Model file for the job. Use its own axes, mm. A direction names the side the tool comes from. Round coordinates to 2 decimals unless told otherwise and drop trailing zeros. Order: outer loops, then holes, each group sorted by start corner. A loop starts at its lowest first (then second) coordinate and runs counter-clockwise, first axis right, second up. Notation, with made-up numbers: (61.25, 68.25) - (120.25, 68.25) arc R18 cw to (120.25, 76.25) - close; hole circle Ø9 at (-37.75, -4.75). An arc over 180 degrees is marked (long way). Put each result on its own line as item: value. Start each with the question number.
Item 1: Which spindle directions (+Z, -Z, +X, -X, +Y, -Y) get a long thin tool onto all of the face, cutting with end or side? Do faces 1 (the face through (2, 0, -0.825)), 2 (the face through (-2.383, -9.777, 8.635)), 3 (the face through (6.95, 2.82, 11.14)), 4 (the face through (7.675, 6.509, 8.635)). Say none if no direction does.
Item 2: Mould opens along Y. For faces 5 (the face through (40.293, -8.948, -11.765)), 6 (the face through (-1, 10, 13.018)), 7 (the face through (0, 0, 5.398)) say: pulls with the +Y half, pulls with the -Y half, needs draft (parallel to the pull), parting line crosses it, or undercut.
Item 3: Probe probe 1 along Y at (x, z) = (0, 8.2); probe 2 along Y at (x, z) = (0, -11) (3 decimals); probe 3 along Z at (x, y) = (-32, 22). List the from-to ranges inside material, lowest first.
Item 4: Saw through at A-A on z = 10.5. List the corners of the cut face in (x, y).
Item 5: Pin check, flat tips, straight feed: pin 1 Ø1.9 at (x, y) = (-1.5, -6) entering from +Z; pin 2 Ø3.5 at (x, y) = (-11, -5.5) entering from +Z; pin 3 Ø1.5 at (x, y) = (-2, 1) entering from -Z; pin 4 Ø4 at (x, z) = (-19, -6.5) entering from +Y. Stop position of each tip, or through.
```python
from build123d import *

# Parameters (mm, degrees)
SKETCH11_R                      = 3.3672
CUT_EXTRUDE5_DEPTH              = 3.81
SKETCH11_5_R                    = 3.3672
CUT_EXTRUDE7_DEPTH              = 7.62
CUT_EXTRUDE8_DEPTH              = 10.16
SKETCH13_R                      = 6.35
CUT_EXTRUDE10_DEPTH             = 12.192
CHAMFER1_SIZE                   = 3.81
CHAMFER2_SIZE                   = 3.81
CUT_EXTRUDE11_DEPTH             = 8.89
F_3_32_0_09375_DIAMETER_HOLE1_D = 2.38125


with BuildPart() as part:
    # Sketch2 → Revolve1 (revolve)
    with BuildSketch(Plane(origin=(0, 0, 0), x_dir=(0, 0, -1), z_dir=(1, 0, 0))):
        Polygon((-13.0175, 0), (-13.0175, 9.525), (-13.0175, 12.7), (-9.8425, 12.7), (10.4775, 12.7), (10.4775, 41.275), (13.0175, 41.275), (13.0175, 0), align=None)
    revolve(axis=Axis((0, 0, -13.0175), (0, 0, 1)))

    # Sketch11 → Cut-Extrude5 (cut)
    with BuildSketch(Plane.XY.offset(13.0175)):
        with BuildLine():
            ThreePointArc((-4.819494332, -5.746518457), (-1.340267005, -7.379273972), (2.490906416, -7.074276304))
            ThreePointArc((2.490906416, -7.074276304), (1.265901972, -5.744591723), (0.392647765, -4.16151748))
            ThreePointArc((0.392647765, -4.16151748), (-0.746975478, -4.11271536), (-1.830973459, -3.757650355))
            ThreePointArc((-1.830973459, -3.757650355), (-3.205144168, -4.932534109), (-4.819494332, -5.746518457))
        make_face()
        with BuildLine():
            ThreePointArc((7.5, 0), (6.796918695, 3.17047256), (4.819494332, 5.746518457))
            ThreePointArc((4.819494332, 5.746518457), (3.205144168, 4.932534109), (1.830973459, 3.757650355))
            ThreePointArc((1.830973459, 3.757650355), (0.746975478, 4.11271536), (-0.392647765, 4.16151748))
            ThreePointArc((-0.392647765, 4.16151748), (-1.265901972, 5.744591723), (-2.490906416, 7.074276304))
            ThreePointArc((-2.490906416, 7.074276304), (-7.379273972, 1.340267005), (-4.819494332, -5.746518457))
            ThreePointArc((-4.819494332, -5.746518457), (-3.205144168, -4.932534109), (-1.830973459, -3.757650355))
            ThreePointArc((-1.830973459, -3.757650355), (-0.746975478, -4.11271536), (0.392647765, -4.16151748))
            ThreePointArc((0.392647765, -4.16151748), (1.265901972, -5.744591723), (2.490906416, -7.074276304))
            ThreePointArc((2.490906416, -7.074276304), (6.120939394, -4.334062868), (7.5, 0))
        make_face()
        Circle(SKETCH11_R, mode=Mode.SUBTRACT)
        Circle(SKETCH11_R)
        with BuildLine():
            ThreePointArc((1.830973459, 3.757650355), (3.205144168, 4.932534109), (4.819494332, 5.746518457))
            ThreePointArc((4.819494332, 5.746518457), (1.340267005, 7.379273972), (-2.490906416, 7.074276304))
            ThreePointArc((-2.490906416, 7.074276304), (-1.265901972, 5.744591723), (-0.392647765, 4.16151748))
            ThreePointArc((-0.392647765, 4.16151748), (0.746975478, 4.11271536), (1.830973459, 3.757650355))
        make_face()
    extrude(amount=-CUT_EXTRUDE5_DEPTH, mode=Mode.SUBTRACT)

    # Sketch11<5> → Cut-Extrude7 (cut)
    with BuildSketch(Plane.XY.offset(13.0175)):
        Circle(SKETCH11_5_R)
    extrude(amount=-CUT_EXTRUDE7_DEPTH, mode=Mode.SUBTRACT)

    # Sketch11<6> → Cut-Extrude8 (cut)
    with BuildSketch(Plane.XY.offset(13.0175)):
        with BuildLine():
            ThreePointArc((-4.819494332, -5.746518457), (-1.340267005, -7.379273972), (2.490906416, -7.074276304))
            ThreePointArc((2.490906416, -7.074276304), (1.265901972, -5.744591723), (0.392647765, -4.16151748))
            ThreePointArc((0.392647765, -4.16151748), (-0.746975478, -4.11271536), (-1.830973459, -3.757650355))
            ThreePointArc((-1.830973459, -3.757650355), (-3.205144168, -4.932534109), (-4.819494332, -5.746518457))
        make_face()
        with BuildLine():
            ThreePointArc((1.830973459, 3.757650355), (3.205144168, 4.932534109), (4.819494332, 5.746518457))
            ThreePointArc((4.819494332, 5.746518457), (1.340267005, 7.379273972), (-2.490906416, 7.074276304))
            ThreePointArc((-2.490906416, 7.074276304), (-1.265901972, 5.744591723), (-0.392647765, 4.16151748))
            ThreePointArc((-0.392647765, 4.16151748), (0.746975478, 4.11271536), (1.830973459, 3.757650355))
        make_face()
    extrude(amount=-CUT_EXTRUDE8_DEPTH, mode=Mode.SUBTRACT)

    # Sketch13 → Cut-Extrude10 (cut)
    with BuildSketch(Plane(origin=(0, 0, -13.0175), x_dir=(-1, 0, 0), z_dir=(0, 0, -1))):
        Circle(SKETCH13_R)
    extrude(amount=-CUT_EXTRUDE10_DEPTH, mode=Mode.SUBTRACT)

    # Chamfer1
    chamfer1_edges = [part.edges().sort_by_distance(p)[0] for p in [
        (6.35, 0, -0.8255),
    ]]
    chamfer(chamfer1_edges, length=CHAMFER1_SIZE)

    # Chamfer2
    chamfer2_edges = [part.edges().sort_by_distance(p)[0] for p in [
        (0, -12.7, -10.4775),
    ]]
    chamfer(chamfer2_edges, length=CHAMFER2_SIZE)

    # Sketch14 → Cut-Extrude11 (cut)
    with BuildSketch(Plane.XY.offset(13.0175)):
        with BuildLine():
            Line((-7.478864421, -0.562660625), (-12.664210419, -0.952771992))
            ThreePointArc((-12.664210419, -0.952771992), (-11.749957105, -4.819596251), (-9.685536123, -8.214644849))
            Line((-9.685536123, -8.214644849), (-5.719804797, -4.851168218))
            ThreePointArc((-5.719804797, -4.851168218), (-6.938951046, -2.846218259), (-7.478864421, -0.562660625))
        make_face()
        with BuildLine():
            ThreePointArc((-4.819596251, 11.749957105), (-8.214644849, 9.685536123), (-10.805586775, 6.673027383))
            Line((-10.805586775, 6.673027383), (-6.381252032, 3.940764202))
            ThreePointArc((-6.381252032, 3.940764202), (-4.851168218, 5.719804797), (-2.846218259, 6.938951046))
            Line((-2.846218259, 6.938951046), (-4.819596251, 11.749957105))
        make_face()
        with BuildLine():
            ThreePointArc((9.685536123, 8.214644849), (6.673027383, 10.805586775), (3.007316228, 12.33880258))
            Line((3.007316228, 12.33880258), (1.775974151, 7.286694437))
            ThreePointArc((1.775974151, 7.286694437), (3.940764202, 6.381252032), (5.719804797, 4.851168218))
            Line((5.719804797, 4.851168218), (9.685536123, 8.214644849))
        make_face()
        with BuildLine():
            Line((6.381252032, -3.940764202), (10.805586775, -6.673027383))
            ThreePointArc((10.805586775, -6.673027383), (12.21722047, -3.468360417), (12.7, 0))
            ThreePointArc((12.7, 0), (12.691049451, 0.476721974), (12.664210419, 0.952771992))
            Line((12.664210419, 0.952771992), (7.478864421, 0.562660625))
            ThreePointArc((7.478864421, 0.562660625), (7.494714243, 0.281528725), (7.5, 0))
            ThreePointArc((7.5, 0), (7.214893979, -2.048244341), (6.381252032, -3.940764202))
        make_face()
        with BuildLine():
            Line((-1.775974151, -7.286694437), (-3.007316228, -12.33880258))
            ThreePointArc((-3.007316228, -12.33880258), (0.952771992, -12.664210419), (4.819596251, -11.749957105))
            Line((4.819596251, -11.749957105), (2.846218259, -6.938951046))
            ThreePointArc((2.846218259, -6.938951046), (0.562660625, -7.478864421), (-1.775974151, -7.286694437))
        make_face()
    extrude(amount=-CUT_EXTRUDE11_DEPTH, mode=Mode.SUBTRACT)

    # 3/32 (0.09375) Diameter Hole1 (through all)
    with Locations(Plane(origin=(1.382526007, -18.376485052, 0), x_dir=(-0.997181923, -0.075021417, 0), z_dir=(0.075021417, -0.997181923, 0))):
        with Locations((0, 0)):
            Hole(F_3_32_0_09375_DIAMETER_HOLE1_D / 2)

    # Sketch17 → Revolve2 (revolve)
    with BuildSketch(Plane(origin=(0, 0, 0), x_dir=(1, 0, 0), z_dir=(0, 1, 0))):
        with BuildLine():
            Line((-41.275, 10.4775), (-39.6875, 10.4775))
            ThreePointArc((-39.6875, 10.4775), (-40.48125, 9.68375), (-41.275, 10.4775))
        make_face()
    revolve(axis=Axis((0, 0, -15.01775), (0, 0, 1)))


solid = part.part
```
Results found:
1. face 1: -Z
1. face 2: +Z, -Y
1. face 3: +Z
1. face 4: +Z, +Y
2. face 5: parting line crosses it
2. face 6: needs draft
2. face 7: undercut
3. probe 1: y = -4.18 to -3.37, 3.37 to 4.18, 7.5 to 12.7
3. probe 2: y = -41.275 to -6.35, 6.35 to 41.275
3. probe 3: z = -13.02 to -10.48
4. outline: (-12.66, -0.95) - (-7.48, -0.56) arc R7.5 cw to (-6.38, 3.94) - (-10.81, 6.67) arc R12.7 ccw to start; (-9.69, -8.21) arc R12.7 ccw to (-3.01, -12.34) - (-1.78, -7.29) arc R7.5 cw to (-5.72, -4.85) - close; (-4.82, 11.75) - (-2.85, 6.94) arc R7.5 cw to (1.78, 7.29) - (3.01, 12.34) arc R12.7 ccw to start; (2.85, -6.94) - (4.82, -11.75) arc R12.7 ccw to (10.81, -6.67) - (6.38, -3.94) arc R7.5 cw to start; (5.72, 4.85) arc R7.5 cw to (7.48, 0.56) - (12.66, 0.95) arc R12.7 ccw to (9.69, 8.21) - close
5. pin 1: stops at z = 2.86
5. pin 2: stops at z = 4.13
5. pin 3: stops at z = -1.27
5. pin 4: passes through
